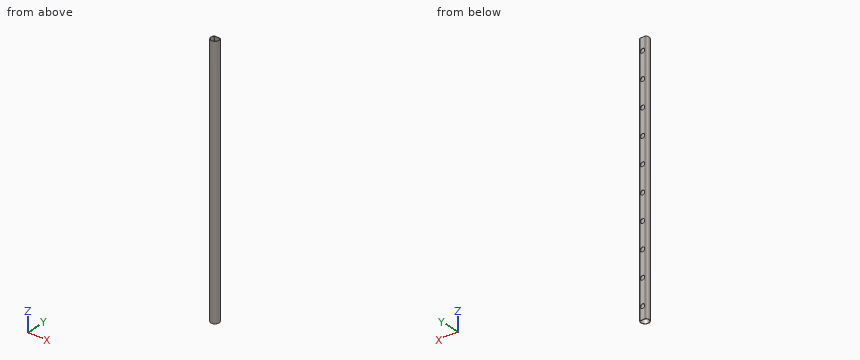
```python
from build123d import *

# Parameters (mm, degrees)
BOSS_EXTRUDE1_DEPTH = 936
CUT_EXTRUDE1_REACH  = 938.481
SKETCH2_R           = 7.9


with BuildPart() as part:
    # Sketch1 → Boss-Extrude1 (new body)
    with BuildSketch(Plane.XY):
        with BuildLine():
            Line((8.94427191, 11), (-8.94427191, 11))
            ThreePointArc((-8.94427191, 11), (-10.169016781, 10.738612788), (-11.180339887, 10))
            ThreePointArc((-11.180339887, 10), (0, -15), (11.180339887, 10))
            ThreePointArc((11.180339887, 10), (10.169016781, 10.738612788), (8.94427191, 11))
        make_face()
        with BuildLine():
            Line((8.94427191, 9.8), (-8.94427191, 9.8))
            ThreePointArc((-8.94427191, 9.8), (-9.679118833, 9.643167673), (-10.285912696, 9.2))
            ThreePointArc((-10.285912696, 9.2), (0, -13.8), (10.285912696, 9.2))
            ThreePointArc((10.285912696, 9.2), (9.679118833, 9.643167673), (8.94427191, 9.8))
        make_face(mode=Mode.SUBTRACT)
    extrude(amount=BOSS_EXTRUDE1_DEPTH)

    # Sketch2 → Cut-Extrude1 (cut, up to next)
    with BuildSketch(Plane(origin=(0, 11, 0), x_dir=(1, 0, 0), z_dir=(0, 1, 0)), mode=Mode.PRIVATE) as cut_extrude1_sk1:
        with Locations(Location((0, -891, 0), (0, 0, 180))):
            Circle(SKETCH2_R)
    cut_extrude1_tool1 = extrude(cut_extrude1_sk1.sketch, amount=-CUT_EXTRUDE1_REACH, mode=Mode.PRIVATE) & part.part
    # Sketch2 → Cut-Extrude1 (cut, up to next)
    with BuildSketch(Plane(origin=(0, 11, 0), x_dir=(1, 0, 0), z_dir=(0, 1, 0)), mode=Mode.PRIVATE) as cut_extrude1_sk2:
        with Locations(Location((0, -797, 0), (0, 0, 180))):
            Circle(SKETCH2_R)
    cut_extrude1_tool2 = extrude(cut_extrude1_sk2.sketch, amount=-CUT_EXTRUDE1_REACH, mode=Mode.PRIVATE) & part.part
    # Sketch2 → Cut-Extrude1 (cut, up to next)
    with BuildSketch(Plane(origin=(0, 11, 0), x_dir=(1, 0, 0), z_dir=(0, 1, 0)), mode=Mode.PRIVATE) as cut_extrude1_sk3:
        with Locations(Location((0, -703, 0), (0, 0, 180))):
            Circle(SKETCH2_R)
    cut_extrude1_tool3 = extrude(cut_extrude1_sk3.sketch, amount=-CUT_EXTRUDE1_REACH, mode=Mode.PRIVATE) & part.part
    # Sketch2 → Cut-Extrude1 (cut, up to next)
    with BuildSketch(Plane(origin=(0, 11, 0), x_dir=(1, 0, 0), z_dir=(0, 1, 0)), mode=Mode.PRIVATE) as cut_extrude1_sk4:
        with Locations(Location((0, -609, 0), (0, 0, 180))):
            Circle(SKETCH2_R)
    cut_extrude1_tool4 = extrude(cut_extrude1_sk4.sketch, amount=-CUT_EXTRUDE1_REACH, mode=Mode.PRIVATE) & part.part
    # Sketch2 → Cut-Extrude1 (cut, up to next)
    with BuildSketch(Plane(origin=(0, 11, 0), x_dir=(1, 0, 0), z_dir=(0, 1, 0)), mode=Mode.PRIVATE) as cut_extrude1_sk5:
        with Locations(Location((0, -515, 0), (0, 0, 180))):
            Circle(SKETCH2_R)
    cut_extrude1_tool5 = extrude(cut_extrude1_sk5.sketch, amount=-CUT_EXTRUDE1_REACH, mode=Mode.PRIVATE) & part.part
    # Sketch2 → Cut-Extrude1 (cut, up to next)
    with BuildSketch(Plane(origin=(0, 11, 0), x_dir=(1, 0, 0), z_dir=(0, 1, 0)), mode=Mode.PRIVATE) as cut_extrude1_sk6:
        with Locations(Location((0, -421, 0), (0, 0, 180))):
            Circle(SKETCH2_R)
    cut_extrude1_tool6 = extrude(cut_extrude1_sk6.sketch, amount=-CUT_EXTRUDE1_REACH, mode=Mode.PRIVATE) & part.part
    # Sketch2 → Cut-Extrude1 (cut, up to next)
    with BuildSketch(Plane(origin=(0, 11, 0), x_dir=(1, 0, 0), z_dir=(0, 1, 0)), mode=Mode.PRIVATE) as cut_extrude1_sk7:
        with Locations(Location((0, -327, 0), (0, 0, 180))):
            Circle(SKETCH2_R)
    cut_extrude1_tool7 = extrude(cut_extrude1_sk7.sketch, amount=-CUT_EXTRUDE1_REACH, mode=Mode.PRIVATE) & part.part
    # Sketch2 → Cut-Extrude1 (cut, up to next)
    with BuildSketch(Plane(origin=(0, 11, 0), x_dir=(1, 0, 0), z_dir=(0, 1, 0)), mode=Mode.PRIVATE) as cut_extrude1_sk8:
        with Locations(Location((0, -233, 0), (0, 0, 180))):
            Circle(SKETCH2_R)
    cut_extrude1_tool8 = extrude(cut_extrude1_sk8.sketch, amount=-CUT_EXTRUDE1_REACH, mode=Mode.PRIVATE) & part.part
    # Sketch2 → Cut-Extrude1 (cut, up to next)
    with BuildSketch(Plane(origin=(0, 11, 0), x_dir=(1, 0, 0), z_dir=(0, 1, 0)), mode=Mode.PRIVATE) as cut_extrude1_sk9:
        with Locations(Location((0, -139, 0), (0, 0, 180))):
            Circle(SKETCH2_R)
    cut_extrude1_tool9 = extrude(cut_extrude1_sk9.sketch, amount=-CUT_EXTRUDE1_REACH, mode=Mode.PRIVATE) & part.part
    # Sketch2 → Cut-Extrude1 (cut, up to next)
    with BuildSketch(Plane(origin=(0, 11, 0), x_dir=(1, 0, 0), z_dir=(0, 1, 0)), mode=Mode.PRIVATE) as cut_extrude1_sk10:
        with Locations(Location((0, -45, 0), (0, 0, 180))):
            Circle(SKETCH2_R)
    cut_extrude1_tool10 = extrude(cut_extrude1_sk10.sketch, amount=-CUT_EXTRUDE1_REACH, mode=Mode.PRIVATE) & part.part
    add(cut_extrude1_tool1.solids().sort_by_distance((0, 11, 891))[0], mode=Mode.SUBTRACT)
    add(cut_extrude1_tool2.solids().sort_by_distance((0, 11, 797))[0], mode=Mode.SUBTRACT)
    add(cut_extrude1_tool3.solids().sort_by_distance((0, 11, 703))[0], mode=Mode.SUBTRACT)
    add(cut_extrude1_tool4.solids().sort_by_distance((0, 11, 609))[0], mode=Mode.SUBTRACT)
    add(cut_extrude1_tool5.solids().sort_by_distance((0, 11, 515))[0], mode=Mode.SUBTRACT)
    add(cut_extrude1_tool6.solids().sort_by_distance((0, 11, 421))[0], mode=Mode.SUBTRACT)
    add(cut_extrude1_tool7.solids().sort_by_distance((0, 11, 327))[0], mode=Mode.SUBTRACT)
    add(cut_extrude1_tool8.solids().sort_by_distance((0, 11, 233))[0], mode=Mode.SUBTRACT)
    add(cut_extrude1_tool9.solids().sort_by_distance((0, 11, 139))[0], mode=Mode.SUBTRACT)
    add(cut_extrude1_tool10.solids().sort_by_distance((0, 11, 45))[0], mode=Mode.SUBTRACT)


solid = part.part
```
The model under review builds one solid part; all positions refer to its coordinate system, in mm. Coordinates: 2 decimals unless noted, no trailing zeros. Write each loop counter-clockwise with the first axis right and the second up, starting at its lowest first coordinate (ties: lowest second). Pieces come first, ordered by that corner, then holes. Notation, with made-up numbers: (-20.75, 29) -> (5.25, 29) arc R6 ccw to (5.25, 40) -> close; hole circle Ø11 at (46, 70). An arc over 180 degrees is marked (long way). One line per item, written item: value. Start each with the question number.
Q1. To check wall thickness, follow probe 1 along Y at (x, z) = (-2, 380.5); probe 2 along X at (y, z) = (1.75, 789.5); probe 3 along X at (y, z) = (0, 284.5). State the ranges of each line that lie inside material, in increasing order.
Q2. Add section B-B, the plane z = 275.5. Give the boundary of the cut face in (x, y), then the cut area to 3 significant figures.
Q3. Clearance check with flat-ended pins moving along their axes: P1, Ø10, axis at y = 0.5, z = 237, coming from the +X side; P2, Ø5, axis at y = -7.5, z = 433, coming from the -X side; P3, Ø2, axis at y = -6, z = 611.5, coming from the +X side; P4, Ø12.5, axis at x = 0, z = 609, coming from the +Y side. State where each tip first meets the part, or that it passes through.
Q4. Add section A-A, the plane y = -9.25. Give the boundary of the cut face in (x, z).
Q5. Add section C-C, the plane x = 0.25. Count the separate pieces of the cut face and the enclosed holes in it, then the cut area to 3 significant figures.
Response:
1. probe 1: -14.87 to -13.65, 9.8 to 11
1. probe 2: -14.9 to -13.69, 13.69 to 14.9
1. probe 3: -15 to -13.8, 13.8 to 15
2. outline: (-11.18, 10) arc R15 ccw (long way) to (11.18, 10) arc R3 ccw to (8.94, 11) -> (-8.94, 11) arc R3 ccw to start; hole (-10.29, 9.2) arc R13.8 ccw (long way) to (10.29, 9.2) arc R1.8 ccw to (8.94, 9.8) -> (-8.94, 9.8) arc R1.8 ccw to start
2. area: 106 mm²
3. P1: x = 15
3. P2: x = -14.14
3. P3: x = 14.14
3. P4: y = -12.3
4. outline: (-11.81, 0) -> (-10.24, 0) -> (-10.24, 936) -> (-11.81, 936) -> close; (10.24, 0) -> (11.81, 0) -> (11.81, 936) -> (10.24, 936) -> close
5. separate pieces: 12
5. enclosed holes: 0
5. area: 2,060 mm²
